Check sheet for the modelled part. Datum: model origin and axes. Units: mm. A direction names the side the tool comes from. Give positions to 0.01 mm unless a question says otherwise; leave off trailing zeros. Loops run counter-clockwise (first coordinate to the right, second up) from the corner with the lowest first, then second, coordinate; pieces in that order, holes last. Notation, with made-up numbers: (-25.75, 50.25) - (32.25, 50.25) arc R17 cw to (32.25, 66.25) - close; hole circle Ø6 at (14, 56.5). An arc over 180 degrees is marked (long way). Use one line per item in the form item = value.
from build123d import *

# Parameters (mm, degrees)
BOSS_EXTRUDE1_DEPTH  = 17.5
CUT_EXTRUDE1_DEPTH   = 15.5
FILLET2_R            = 1.5
CUT_EXTRUDE4_REACH   = 46.612
SKETCH5_W            = 11
SKETCH5_H            = 2.5
CUT_EXTRUDE5_REACH   = 46.612
SKETCH6_W            = 11
SKETCH6_H            = 2.5
CUT_EXTRUDE6_DEPTH   = 1
BOSS_EXTRUDE7_DEPTH  = 8.5
SKETCH3_11_R         = 1
BOSS_EXTRUDE8_DEPTH  = 6
CUT_EXTRUDE8_REACH   = 38.949
SKETCH3_12_W         = 13
SKETCH3_12_H         = 16.5
BOSS_EXTRUDE9_DEPTH  = 8.5
CUT_EXTRUDE9_REACH   = 57.057
SKETCH11_W           = 25
SKETCH11_H           = 45
SKETCH11_W_2         = 13
SKETCH11_H_2         = 16.5
BOSS_EXTRUDE10_DEPTH = 0.5
CHAMFER1_SIZE        = 1
FILLET3_R            = 1


with BuildPart() as part:
    # Sketch1 → Boss-Extrude1 (new body)
    with BuildSketch(Plane(origin=(0, 0, 0), x_dir=(1, 0, 0), z_dir=(0, 1, 0))):
        Polygon((-15, 20), (15, 20), (15, -20), (15, -30), (-15, -30), (-15, -20), align=None)
    extrude(amount=BOSS_EXTRUDE1_DEPTH)

    # Sketch2 → Cut-Extrude1 (cut)
    with BuildSketch(Plane(origin=(0, 17.5, 0), x_dir=(1, 0, 0), z_dir=(0, 1, 0))):
        Polygon((-13, 18), (13, 18), (13, -18), (13, -28), (-13, -28), (-13, -18), align=None)
    extrude(amount=-CUT_EXTRUDE1_DEPTH, mode=Mode.SUBTRACT)

    # Fillet2
    fillet2_edges = [part.edges().sort_by_distance(p)[0] for p in [
        (15, 8.75, 30),
        (-15, 8.75, 30),
        (-15, 8.75, -20),
        (15, 8.75, -20),
        (0, 0, 30),
        (-15, 0, 5),
        (0, 0, -20),
        (15, 0, 5),
    ]]
    fillet(fillet2_edges, radius=FILLET2_R)

    # Sketch5 → Cut-Extrude4 (cut, up to next)
    with BuildSketch(Plane.ZY.offset(-13), mode=Mode.PRIVATE) as cut_extrude4_sk1:
        with Locations((17.5, 13.25)):
            Rectangle(SKETCH5_W, SKETCH5_H)
    cut_extrude4_tool1 = extrude(cut_extrude4_sk1.sketch, amount=-CUT_EXTRUDE4_REACH, mode=Mode.PRIVATE) & part.part
    add(cut_extrude4_tool1.solids().sort_by_distance((13, 13.25, 17.5))[0], mode=Mode.SUBTRACT)

    # Sketch6 → Cut-Extrude5 (cut, up to next)
    with BuildSketch(Plane(origin=(-13, 0, 0), x_dir=(0, 0, -1), z_dir=(1, 0, 0)), mode=Mode.PRIVATE) as cut_extrude5_sk1:
        with Locations((7.5, 13.25)):
            Rectangle(SKETCH6_W, SKETCH6_H)
    cut_extrude5_tool1 = extrude(cut_extrude5_sk1.sketch, amount=-CUT_EXTRUDE5_REACH, mode=Mode.PRIVATE) & part.part
    add(cut_extrude5_tool1.solids().sort_by_distance((-13, 13.25, -7.5))[0], mode=Mode.SUBTRACT)

    # Sketch7 → Cut-Extrude6 (cut)
    with BuildSketch(Plane(origin=(0, 17.5, 0), x_dir=(1, 0, 0), z_dir=(0, 1, 0))):
        Polygon((-13, 18), (-14, 18), (-14, -19), (-14, -29), (14, -29), (14, -19), (14, 18), (13, 18), (13, -18), (13, -28), (-13, -28), (-13, -18), align=None)
    extrude(amount=-CUT_EXTRUDE6_DEPTH, mode=Mode.SUBTRACT)

    # Sketch3 → Boss-Extrude7 (add)
    with BuildSketch(Plane(origin=(0, 2, 0), x_dir=(1, 0, 0), z_dir=(0, 1, 0))):
        Polygon((-7.5, -2.505360959), (-7.5, -1.505360959), (-7.5, 18), (-13, 18), (-13, -18), (-7.5, -18), (-7.5, -6.505360959), align=None)
        Polygon((7.5, -2.505360959), (7.5, -3.505360959), (7.5, -6.505360959), (7.5, -9.752680479), (7.5, -18), (13, -18), (13, 18), (7.5, 18), (7.5, -1.505360959), align=None)
    extrude(amount=BOSS_EXTRUDE7_DEPTH)

    # Sketch3<11> → Boss-Extrude8 (add)
    # profile 1 of 3: a face of its own
    with BuildSketch(Plane(origin=(0, 2, 0), x_dir=(1, 0, 0), z_dir=(0, 1, 0))):
        Polygon((1.5, -1.505360959), (-6.5, -1.505360959), (-7.5, -1.505360959), (-7.5, -2.505360959), (-7.5, -6.505360959), (-7.5, -18), (-1.5, -18), (1.5, -18), (7.5, -18), (7.5, -9.752680479), (1.5, -9.752680479), (1.5, -3.505360959), align=None)
        with Locations(Location((0, -4.505360959, 0), (0, 0, 270))):
            Circle(SKETCH3_11_R, mode=Mode.SUBTRACT)
    # profile 2 of 3: a face of its own
    with BuildSketch(Plane(origin=(0, 2, 0), x_dir=(1, 0, 0), z_dir=(0, 1, 0))):
        Polygon((-7.5, -1.505360959), (-6.5, -1.505360959), (-6.5, 14.994639041), (6.5, 14.994639041), (6.5, -1.505360959), (7.5, -1.505360959), (7.5, 18), (-7.5, 18), align=None)
    # profile 3 of 3: a face of its own
    with BuildSketch(Plane(origin=(0, 2, 0), x_dir=(1, 0, 0), z_dir=(0, 1, 0))):
        Polygon((6.214337826, -1.505360959), (1.5, -1.505360959), (1.5, -3.505360959), (7.5, -3.505360959), (7.5, -2.505360959), (7.5, -1.505360959), (6.5, -1.505360959), align=None)
    extrude(amount=BOSS_EXTRUDE8_DEPTH)

    # Sketch3<12> → Cut-Extrude8 (cut, up to next)
    with BuildSketch(Plane(origin=(0, 2, 0), x_dir=(1, 0, 0), z_dir=(0, 1, 0)), mode=Mode.PRIVATE) as cut_extrude8_sk1:
        with Locations((0, 6.744639041)):
            Rectangle(SKETCH3_12_W, SKETCH3_12_H)
    cut_extrude8_tool1 = extrude(cut_extrude8_sk1.sketch, amount=-CUT_EXTRUDE8_REACH, mode=Mode.PRIVATE) & part.part
    add(cut_extrude8_tool1.solids().sort_by_distance((0, 2, -6.744639))[0], mode=Mode.SUBTRACT)

    # Sketch3<13> → Boss-Extrude9 (add)
    with BuildSketch(Plane(origin=(0, 2, 0), x_dir=(1, 0, 0), z_dir=(0, 1, 0))):
        Polygon((-7.5, -18), (-13, -18), (-13, -20), (13, -20), (13, -18), (7.5, -18), (1.5, -18), (-1.5, -18), align=None)
    extrude(amount=BOSS_EXTRUDE9_DEPTH)

    # Sketch10 → Cut-Extrude9 (cut, up to next)
    with BuildSketch(Plane.XY.offset(30), mode=Mode.PRIVATE) as cut_extrude9_sk1:
        with BuildLine():
            Line((-3, 17.5), (3, 17.5))
            ThreePointArc((3, 17.5), (0, 14.5), (-3, 17.5))
        make_face()
    cut_extrude9_tool1 = extrude(cut_extrude9_sk1.sketch, amount=-CUT_EXTRUDE9_REACH, mode=Mode.PRIVATE) & part.part
    add(cut_extrude9_tool1.solids().sort_by_distance((0, 16.22676, 30))[0], mode=Mode.SUBTRACT)

    # Sketch11 → Boss-Extrude10 (add)
    with BuildSketch(Plane.XZ):
        with Locations((0, 5)):
            Rectangle(SKETCH11_W, SKETCH11_H)
        with Locations((0, -6.744639041)):
            Rectangle(SKETCH11_W_2, SKETCH11_H_2, mode=Mode.SUBTRACT)
    extrude(amount=BOSS_EXTRUDE10_DEPTH)

    # Chamfer1
    # the kernel refuses this chamfer: 1 mm, written as the material it takes off along each edge
    with BuildSketch(Plane(origin=(-15.071682988, -0.5, 27.5), x_dir=(0, -0.027495876610586403, -0.9996219169112968), z_dir=(1, 0, 0))) as chamfer1_piece_1_section:
        Polygon((CHAMFER1_SIZE * 0.999621916911, CHAMFER1_SIZE * 0.0274958766106), (-CHAMFER1_SIZE * 0.0274958766106, CHAMFER1_SIZE * 0.999621916911), (0, 0), align=None)
    chamfer1_piece_1 = extrude(amount=30.143365976, mode=Mode.PRIVATE)
    chamfer1_piece_1 = split(chamfer1_piece_1, bisect_by=Plane(origin=(0, 0, 27.106598916), z_dir=(0, -1, 0)), keep=Keep.TOP, mode=Mode.PRIVATE)
    add(chamfer1_piece_1, mode=Mode.SUBTRACT)
    with BuildSketch(Plane(origin=(-12.5, -0.5, -20.071682988), x_dir=(0.9996219169112968, -0.027495876610586403, 0), z_dir=(0, 0, 1))) as chamfer1_piece_2_section:
        Polygon((CHAMFER1_SIZE * 0.999621916911, CHAMFER1_SIZE * 0.0274958766106), (-CHAMFER1_SIZE * 0.0274958766106, CHAMFER1_SIZE * 0.999621916911), (0, 0), align=None)
    chamfer1_piece_2 = extrude(amount=50.143365976, mode=Mode.PRIVATE)
    chamfer1_piece_2 = split(chamfer1_piece_2, bisect_by=Plane(origin=(-12.106598916, 0, 5), z_dir=(0, -1, 0)), keep=Keep.TOP, mode=Mode.PRIVATE)
    add(chamfer1_piece_2, mode=Mode.SUBTRACT)
    with BuildSketch(Plane(origin=(12.5, -0.5, 30.071682988), x_dir=(-0.9996219169112968, -0.027495876610586403, 0), z_dir=(0, 0, -1))) as chamfer1_piece_3_section:
        Polygon((CHAMFER1_SIZE * 0.999621916911, CHAMFER1_SIZE * 0.0274958766106), (-CHAMFER1_SIZE * 0.0274958766106, CHAMFER1_SIZE * 0.999621916911), (0, 0), align=None)
    chamfer1_piece_3 = extrude(amount=50.143365976, mode=Mode.PRIVATE)
    chamfer1_piece_3 = split(chamfer1_piece_3, bisect_by=Plane(origin=(12.106598916, 0, 5), z_dir=(0, -1, 0)), keep=Keep.TOP, mode=Mode.PRIVATE)
    add(chamfer1_piece_3, mode=Mode.SUBTRACT)
    with BuildSketch(Plane(origin=(15.071682988, -0.5, -17.5), x_dir=(0, -0.027495876610586403, 0.9996219169112968), z_dir=(-1, 0, 0))) as chamfer1_piece_4_section:
        Polygon((CHAMFER1_SIZE * 0.999621916911, CHAMFER1_SIZE * 0.0274958766106), (-CHAMFER1_SIZE * 0.0274958766106, CHAMFER1_SIZE * 0.999621916911), (0, 0), align=None)
    chamfer1_piece_4 = extrude(amount=30.143365976, mode=Mode.PRIVATE)
    chamfer1_piece_4 = split(chamfer1_piece_4, bisect_by=Plane(origin=(0, 0, -17.106598916), z_dir=(0, -1, 0)), keep=Keep.TOP, mode=Mode.PRIVATE)
    add(chamfer1_piece_4, mode=Mode.SUBTRACT)

    # Fillet3
    fillet3_edges = [part.edges().sort_by_distance(p)[0] for p in [
        (1.5, 2, 6.629020719),
        (0, 2, 20),
    ]]
    fillet(fillet3_edges, radius=FILLET3_R)


solid = part.part
Item 1: Section check D-D on y = 9.5. Record the boundary of the cut face in (x, z).
Answer block:
outline = (-15, -18.5) arc R1.5 ccw to (-13.5, -20) - (13.5, -20) arc R1.5 ccw to (15, -18.5) - (15, 28.5) arc R1.5 ccw to (13.5, 30) - (-13.5, 30) arc R1.5 ccw to (-15, 28.5) - close; hole (-13, 20) - (13, 20) - (13, 28) - (-13, 28) - close; hole (-7.5, -18) - (7.5, -18) - (7.5, 18) - (-7.5, 18) - close
Item 2: Section check B-B on x = 0. Record the boundary of the cut face in (y, z), then the cut area to 3 significant figures.
Answer block:
outline = (-0.5, -16.5) - (0, -17) - (0, -18.5) arc R1.5 ccw to (1.5, -20) - (17.5, -20) - (17.5, -18) - (8, -18) - (8, -14.99) - (-0.5, -14.99) - close; (-0.5, 1.51) - (8, 1.51) - (8, 3.51) - (2, 3.51) - (2, 5.51) - (8, 5.51) - (8, 18) - (10.5, 18) - (10.5, 20) - (3, 20) arc R1 cw to (2, 21) - (2, 28) - (14.5, 28) - (14.5, 30) - (1.5, 30) arc R1.5 ccw to (0, 28.5) - (0, 27) - (-0.5, 26.5) - close
area = 258 mm2
Item 3: Mould release check, pull along X, two halves, no side actions. Record for faces 4 (the face through (-0.19, 0.43, 29.55)), 5 (the face through (-0.38, 4.96, 5.43)), 6 (the face through (-15, 9, 5)), 7 (the face through (0, 7, 20)): released by +X, released by -X, zero draft, split by the parting line, or undercut.
Answer block:
face_4 = zero draft
face_5 = undercut
face_6 = released by -X
face_7 = undercut
Item 4: Gauge pin test, flat ends, axial feed: P1, Ø7.5, axis at x = 5, z = 23, coming from the +Y side; P2, Ø0.6, axis at x = -14, y = 13.5, coming from the -Z side; P3, Ø1, axis at x = 14, z = 18.5, coming from the -Y side. Record the tip position at first contact, or that the pin passes through.
Answer block:
P1 = 10.5
P2 = -19.99
P3 = 0
Item 5: Thickness scan on L1, parallel to Z at x = 1.25, y = 5; L2, parallel to X at y = 13.25, z = 5.5; L3, parallel to X at y = 5.75, z = 6.5. Record the ranges inside material, lowest first.
Answer block:
L1 = -20 to -14.99, 1.51 to 20, 28 to 30
L2 = -15 to -13, 13 to 15
L3 = -15 to 1.5, 7.5 to 15
Item 6: Access from +Z, -Z, +X, -X, +Y, -Y to the whole of each face (thin tool, end or side, straight path). Record for faces 1 (the face through (14, 17, 6)), 2 (the face through (0.1, 14.5, 29)), 3 (the face through (6.5, 4, -7)).
Answer block:
face_1 = +Y
face_2 = +Z, +Y
face_3 = +Y, -Y
Item 7: Section check A-A on z = -9.5. Give the number of separate pieces and of enclosed holes in the cut face, then the cut area to 3 significant figures.
Answer block:
separate_pieces = 3
enclosed_holes = 0
area = 199 mm2
Item 8: Section check C-C on z = 13.5. Record the boundary of the cut face in (x, y), then the cut area to 3 significant figures.
Answer block:
outline = (-15, 1.5) arc R1.5 ccw to (-13.5, 0) - (-12, 0) - (-11.5, -0.5) - (11.5, -0.5) - (12, 0) - (13.5, 0) arc R1.5 ccw to (15, 1.5) - (15, 12) - (13, 12) - (13, 10.5) - (7.5, 10.5) - (7.5, 8) - (-7.5, 8) - (-7.5, 10.5) - (-13, 10.5) - (-13, 16.5) - (-14, 16.5) - (-14, 17.5) - (-15, 17.5) - close; (13, 14.5) - (15, 14.5) - (15, 17.5) - (14, 17.5) - (14, 16.5) - (13, 16.5) - close
area = 309 mm2
